For this review, take the finished solid that the model builds, in its own axes (mm). Face numbers are marked on the shaded views. A direction names the side the tool comes from. Coordinates: 2 decimals unless noted, no trailing zeros. Loops run counter-clockwise (first coordinate to the right, second up) from the corner with the lowest first, then second, coordinate; pieces in that order, holes last. Notation, with made-up numbers: (40, -37) -> (78, -37) arc R32 ccw to (78, -6) -> close; hole circle Ø10 at (18.5, -23). An arc over 180 degrees is marked (long way). Answer in a Markdown table with one row per item.
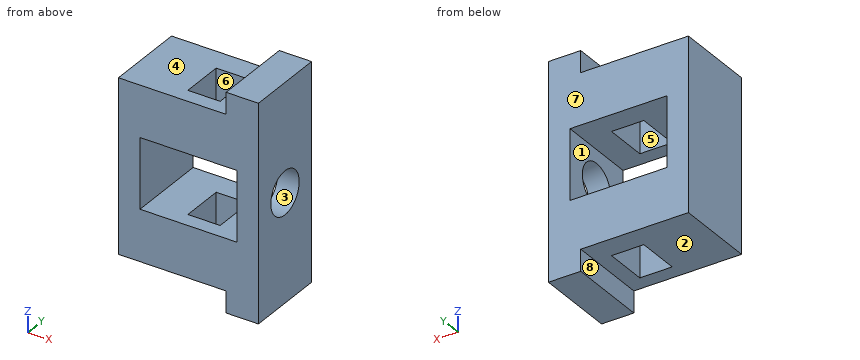
from build123d import *

# Parameters (mm, degrees)
F0_W      = 30
F0_H      = 64
F1_DEPTH  = 52
F2_W      = 36
F2_H      = 26
F3_DEPTH  = 100
F4_W      = 12
F4_H      = 30
F5_DEPTH  = 8
F6_W      = 12
F6_H      = 30
F7_DEPTH  = 8
F8_R      = 8
F9_DEPTH  = 10
F11_W     = 12
F11_H     = 16
F12_DEPTH = 100


with BuildPart() as f1:
    # F0 (on Right) → F1 (new body)
    with BuildSketch(Plane.YZ):
        Rectangle(F0_W, F0_H)
    extrude(amount=F1_DEPTH)

    # F2 (on face) → F3 (cut)
    with BuildSketch(Plane(origin=(0, 15, 0), x_dir=(-1, 0, 0), z_dir=(0, 1, 0))):
        with Locations((-26, 0)):
            Rectangle(F2_W, F2_H)
    extrude(amount=-F3_DEPTH, mode=Mode.SUBTRACT)

    # F4 (on face) → F5 (join)
    with BuildSketch(Plane(origin=(0, 0, -32), x_dir=(1, 0, 0), z_dir=(0, 0, -1))):
        with Locations((46, 0)):
            Rectangle(F4_W, F4_H)
    extrude(amount=F5_DEPTH)

    # F6 (on face) → F7 (join)
    with BuildSketch(Plane.XY.offset(32)):
        with Locations((46, 0)):
            Rectangle(F6_W, F6_H)
    extrude(amount=F7_DEPTH)

    # F8 (on face) → F9 (cut)
    with BuildSketch(Plane.YZ.offset(52)):
        Circle(F8_R)
    extrude(amount=-F9_DEPTH, mode=Mode.SUBTRACT)

    # F11 (on face) → F12 (cut)
    with BuildSketch(Plane.XY.offset(32)):
        with Locations((28.151316, -1.473685)):
            Rectangle(F11_W, F11_H)
    extrude(amount=-F12_DEPTH, mode=Mode.SUBTRACT)


solid = f1.part
Item 1: Take a section at C-C, the plane z = 0. State the section outline as (x, y) points, and give its area (3 significant figures).
Worked answers:
| item | result |
|---|---|
| outline | (0, -15) -> (8, -15) -> (8, 15) -> (0, 15) -> close; (44, -15) -> (52, -15) -> (52, -8) -> (44, -8) -> close; (44, 8) -> (52, 8) -> (52, 15) -> (44, 15) -> close |
| area | 352 mm² |
Item 2: Take a section at A-A, the plane y = -13. State the section outline as (x, z) points, and give its area (3 significant figures).
Worked answers:
| item | result |
|---|---|
| outline | (0, -32) -> (40, -32) -> (40, -40) -> (52, -40) -> (52, 40) -> (40, 40) -> (40, 32) -> (0, 32) -> close; hole (8, -13) -> (44, -13) -> (44, 13) -> (8, 13) -> close |
| area | 2,580 mm² |
Item 3: For L1, parallel to Z at x = 47.25, y = 0; L2, parallel to Z at x = 43, y = -2.5; L3, parallel to X at y = 8.25, z = -3.5, list the stretches that pass through material, from the lowest coordinate up.
Worked answers:
| item | result |
|---|---|
| L1 | -40 to -8, 8 to 40 |
| L2 | -40 to -13, 13 to 40 |
| L3 | 0 to 8, 44 to 52 |
Item 4: Take a section at D-D, the plane z = -16. State the section outline as (x, y) points.
Worked answers:
| item | result |
|---|---|
| outline | (0, -15) -> (52, -15) -> (52, 15) -> (0, 15) -> close; hole (22.15, -9.47) -> (34.15, -9.47) -> (34.15, 6.53) -> (22.15, 6.53) -> close |
Item 5: Take a section at B-B, the plane x = 28. State the section outline as (y, z) points.
Worked answers:
| item | result |
|---|---|
| outline | (-15, -32) -> (-9.47, -32) -> (-9.47, -13) -> (-15, -13) -> close; (-15, 13) -> (-9.47, 13) -> (-9.47, 32) -> (-15, 32) -> close; (6.53, -32) -> (15, -32) -> (15, -13) -> (6.53, -13) -> close; (6.53, 13) -> (15, 13) -> (15, 32) -> (6.53, 32) -> close |
Item 6: Insertion check: pin 1 (5 mm diameter, centred on x = 32.5, y = -6.5, fed in from +Z); pin 2 (8 mm diameter, centred on x = 27, y = 10, fed in from -Z); pin 3 (6.5 mm diameter, centred on y = -1, z = -37.5, fed in from -X); pin 4 (1.5 mm diameter, centred on x = 25, y = -8, fed in from -Z). Each pin has a flat end and moves straight along its axis. Give the tip position at first contact, or say it passes through.
Worked answers:
| item | result |
|---|---|
| pin 1 | z = 32 |
| pin 2 | z = -32 |
| pin 3 | x = 40 |
| pin 4 | through |
Item 7: The part is to be moulded in two halves that separate along Y. For the marked faces 6, 7 and 8, say which applies: +Y half, -Y half, draft (parallel to the pull), parting line (faces both ways), or undercut.
Worked answers:
| item | result |
|---|---|
| face 6 | undercut |
| face 7 | +Y half |
| face 8 | draft |
Item 8: For the marked faces 1, 2, 3, 4 and 5, list the 3-axis set-ups (+Z, -Z, +X, -X, +Y, -Y) from which the entire face can be reached by the end or side of a thin tool; tool diameter is ignored.
Worked answers:
| item | result |
|---|---|
| face 1 | +Y, -Y |
| face 2 | -Z, -X, +Y, -Y |
| face 3 | +X |
| face 4 | +Z, -X, +Y, -Y |
| face 5 | +Z, -Z |
